```python
from build123d import *

# Parameters (mm, degrees)
EXTRUDE_1_DEPTH     = 10
CUT_EXTRUDE_1_DEPTH = 54
CUT_EXTRUDE_2_DEPTH = 54
EXTRUDE_START       = 45
EXTRUDE_2_DEPTH     = 45
CHAMFER_1_SIZE      = 3
EXTRUDE_START_2     = 12
EXTRUDE_3_DEPTH     = 12
CUT_EXTRUDE_4_DEPTH = 12
EXTRUDE_4_DEPTH     = 8
CHAMFER_7_SIZE      = 3
SKETCH_7_R          = 1.3
CUT_EXTRUDE_3_DEPTH = 10
CHAMFER_4_SIZE      = 1
CHAMFER_5_SIZE      = 0.5
CHAMFER_6_SIZE      = 0.5


with BuildPart() as part:
    # 草图1 → 凸台-拉伸1 (new body)
    with BuildSketch(Plane.XY):
        with BuildLine():
            Line((-10, 0), (-19, 0))
            Line((-19, 0), (-19, -6))
            Line((-19, -6), (-13.747727085, -6))
            ThreePointArc((-13.747727085, -6), (-10.799286806, -10.410350834), (-6.5, -13.518505835))
            Line((-6.5, -13.518505835), (-6.5, -29))
            Line((-6.5, -29), (6.5, -29))
            Line((6.5, -29), (6.5, -13.518505835))
            ThreePointArc((6.5, -13.518505835), (10.799286806, -10.410350834), (13.747727085, -6))
            Line((13.747727085, -6), (19, -6))
            Line((19, -6), (19, 0))
            Line((19, 0), (10, 0))
            ThreePointArc((10, 0), (0, -10), (-10, 0))
        make_face()
    extrude(amount=EXTRUDE_1_DEPTH)

    # 草图3 → 切除-拉伸1 (cut)
    with BuildSketch(Plane(origin=(6.5, 0, 0), x_dir=(0, 0, -1), z_dir=(1, 0, 0))):
        with BuildLine():
            Line((-3.86862915, -23.86862915), (-2.7372583, -25))
            Line((-2.7372583, -25), (-3.86862915, -26.13137085))
            ThreePointArc((-3.86862915, -26.13137085), (-6.6, -25), (-3.86862915, -23.86862915))
        make_face()
    extrude(amount=-CUT_EXTRUDE_1_DEPTH, mode=Mode.SUBTRACT)

    # 草图4 → 切除-拉伸2 (cut)
    with BuildSketch(Plane(origin=(0, 0, 0), x_dir=(1, 0, 0), z_dir=(0, 1, 0))):
        with BuildLine():
            Line((-15, -3.161522369), (-15.919238816, -4.080761184))
            ThreePointArc((-15.919238816, -4.080761184), (-15, -6.3), (-14.080761184, -4.080761184))
            Line((-14.080761184, -4.080761184), (-15, -3.161522369))
        make_face()
        with BuildLine():
            Line((15, -3.161522369), (14.080761184, -4.080761184))
            ThreePointArc((14.080761184, -4.080761184), (15, -6.3), (15.919238816, -4.080761184))
            Line((15.919238816, -4.080761184), (15, -3.161522369))
        make_face()
    extrude(amount=-CUT_EXTRUDE_2_DEPTH, mode=Mode.SUBTRACT)

    # 草图5 → 凸台-拉伸2 (add)
    with BuildSketch(Plane(origin=(0, 0, 0), x_dir=(-1, 0, 0), z_dir=(0, 0, -1)).offset(EXTRUDE_START)):
        with BuildLine():
            Line((10, 0), (15, 0))
            ThreePointArc((15, 0), (0, -15), (-15, 0))
            Line((-15, 0), (-10, 0))
            ThreePointArc((-10, 0), (0, -10), (10, 0))
        make_face()
    extrude(amount=-EXTRUDE_2_DEPTH)

    # 倒角1
    chamfer_1_edges = [part.edges().sort_by_distance(p)[0] for p in [
        (0, -29, 0),
        (0, -29, 10),
    ]]
    chamfer(chamfer_1_edges, length=CHAMFER_1_SIZE)

    # 草图8 → 凸台-拉伸3 (add)
    with BuildSketch(Plane(origin=(0, 0, 0), x_dir=(-1, 0, 0), z_dir=(0, 0, -1)).offset(EXTRUDE_START_2)):
        with BuildLine():
            Line((-15, 0), (-19, 0))
            Line((-19, 0), (-19, -6))
            Line((-19, -6), (-13.747727085, -6))
            ThreePointArc((-13.747727085, -6), (-14.683594694, -3.064644655), (-15, 0))
        make_face()
        with BuildLine():
            Line((13.747727085, -6), (19, -6))
            Line((19, -6), (19, 0))
            Line((19, 0), (15, 0))
            ThreePointArc((15, 0), (14.683594694, -3.064644655), (13.747727085, -6))
        make_face()
    extrude(amount=-EXTRUDE_3_DEPTH)

    # 草图9 → 切除-拉伸4 (cut)
    with BuildSketch(Plane(origin=(0, 0, 0), x_dir=(1, 0, 0), z_dir=(0, 1, 0))):
        with BuildLine():
            Line((15, 6.838477631), (14.080761184, 5.919238816))
            ThreePointArc((14.080761184, 5.919238816), (15, 3.7), (15.919238816, 5.919238816))
            Line((15.919238816, 5.919238816), (15, 6.838477631))
        make_face()
        with BuildLine():
            Line((-15, 6.838477631), (-15.919238816, 5.919238816))
            ThreePointArc((-15.919238816, 5.919238816), (-15, 3.7), (-14.080761184, 5.919238816))
            Line((-14.080761184, 5.919238816), (-15, 6.838477631))
        make_face()
    extrude(amount=-CUT_EXTRUDE_4_DEPTH, mode=Mode.SUBTRACT)

    # 草图10 → 凸台-拉伸4 (add)
    with BuildSketch(Plane(origin=(0, 0, -45), x_dir=(-1, 0, 0), z_dir=(0, 0, -1))):
        with BuildLine():
            Line((-15, 0), (-18, 0))
            ThreePointArc((-18, 0), (0, -18), (18, 0))
            Line((18, 0), (15, 0))
            ThreePointArc((15, 0), (0, -15), (-15, 0))
        make_face()
    extrude(amount=-EXTRUDE_4_DEPTH)

    # 倒角7
    chamfer_7_edges = [part.edges().sort_by_distance(p)[0] for p in [
        (0, -15, -37),
    ]]
    chamfer(chamfer_7_edges, length=CHAMFER_7_SIZE - 0.0001)  # a hair under: the kernel refuses the full size

    # 草图7 → 切除-拉伸3 (cut)
    with BuildSketch(Plane(origin=(0, 0, -45), x_dir=(-1, 0, 0), z_dir=(0, 0, -1))):
        with Locations((-9.899494937, -9.899494937)):
            Circle(SKETCH_7_R)
        with Locations(Location((9.899494937, -9.899494937, 0), (0, 0, 180))):
            Circle(SKETCH_7_R)
    extrude(amount=-CUT_EXTRUDE_3_DEPTH, mode=Mode.SUBTRACT)

    # 倒角4
    chamfer_4_edges = [part.edges().sort_by_distance(p)[0] for p in [
        (-19, -3, 10),
        (19, -3, -12),
        (-19, -3, -12),
        (19, -3, 10),
    ]]
    chamfer(chamfer_4_edges, length=CHAMFER_4_SIZE)

    # 倒角5
    chamfer_5_edges = [part.edges().sort_by_distance(p)[0] for p in [
        (-6.5, -25, 6.6),
        (-6.5, -24.434314575, 3.302943725),
        (-6.5, -25.565685425, 3.302943725),
        (6.5, -25, 6.6),
        (6.5, -25.565685425, 3.302943725),
        (6.5, -24.434314575, 3.302943725),
        (0, -10, 10),
        (0, -10, -45),
    ]]
    chamfer(chamfer_5_edges, length=CHAMFER_5_SIZE)

    # 倒角6
    chamfer_6_edges = [part.edges().sort_by_distance(p)[0] for p in [
        (11.199494937, -9.899494937, -35),
        (11.199494937, -9.899494937, -45),
        (-11.199494937, -9.899494937, -35),
        (-11.199494937, -9.899494937, -45),
    ]]
    chamfer(chamfer_6_edges, length=CHAMFER_6_SIZE)


solid = part.part
```
The model under review builds one solid part; all positions refer to its coordinate system, in mm. A direction names the side the tool comes from. Round coordinates to 2 decimals unless told otherwise and drop trailing zeros. Loops run counter-clockwise (first coordinate to the right, second up) from the corner with the lowest first, then second, coordinate; pieces in that order, holes last.
1) Wall thickness on line 1 along X through (y, z) = (-4.5, -5); line 2 along X through (y, z) = (-2, -5); line 3 along X through (y, z) = (-9, 1): over which ranges is each line inside the solid? List them lowest first.
Values follow:
line 1: x = -19 to -16.3, -13.7 to -8.93, 8.93 to 13.7, 16.3 to 19
line 2: x = -19 to -16.3, -13.7 to -9.8, 9.8 to 13.7, 16.3 to 19
line 3: x = -12 to -4.36, 4.36 to 12
2) Tool access review of faces 4 (the face through (6.5, -20, 5)), 5 (the face through (-16, -6, -1)), 6 (the face through (10, -10, -35)): name each direction out of +Z, -Z, +X, -X, +Y, -Y from which nothing blocks a thin tool from reaching the whole face with its end or side.
Values follow:
face 4: +Z, +X, -Y
face 5: +Z, -X, -Y
face 6: -Z
3) Consider section C-C on z = -31. State the section outline as (x, y) points, then the cut area to 3 significant figures.
Values follow:
outline: (-15, 0) arc R15 ccw to (15, 0) - (10, 0) arc R10 cw to (-10, 0) - close
area: 196 mm2
4) Consider section A-A on z = -8. State the section outline as (x, y) points, then the cut area to 3 significant figures.
Values follow:
outline: (-19, -6) - (-13.75, -6) arc R15 ccw to (13.75, -6) - (19, -6) - (19, 0) - (10, 0) arc R10 cw to (-10, 0) - (-19, 0) - close
area: 249 mm2
5) The part is to be moulded in two halves that separate along Y. For faces 1 (the face through (-10.07, -11.19, -40.06)), 2 (the face through (15, -3, -3.7)), 3 (the face through (0.22, -10.14, -44.64)), say which applies: pulls with the +Y half, pulls with the -Y half, needs draft (parallel to the pull), parting line crosses it, or undercut.
Values follow:
face 1: undercut
face 2: needs draft
face 3: pulls with the +Y half
6) Clearance check with flat-ended pins moving along their axes: P1, Ø1.3, axis at x = 9.5, y = -10, coming from the -Z side; P2, Ø4, axis at y = -6.5, z = -24, coming from the +X side; P3, Ø2, axis at x = 9.9, y = -9.9, coming from the -Z side. State where each tip first meets the part, or that it passes through.
Values follow:
P1: stops at z = -35.26
P2: stops at x = 14.31
P3: stops at z = -35.2
7) Consider section B-B on y = -5. Give the number of separate pieces and of enclosed holes in the cut face, then the cut area to 3 significant figures.
Values follow:
separate pieces: 2
enclosed holes: 4
area: 851 mm2
